Design review of the part built by this model. Coordinates are the model's own, in mm. Give positions to 0.01 mm unless a question says otherwise; leave off trailing zeros. Loops run counter-clockwise (first coordinate to the right, second up) from the corner with the lowest first, then second, coordinate; pieces in that order, holes last.
from build123d import *

# Parameters (mm, degrees)
SKETCH_1_R      = 1.6
EXTRUDE_2_DEPTH = 2.5
SKETCH_2_R      = 1.6
EXTRUDE_4_DEPTH = 2.5


with BuildPart() as part:
    # 草图1 → 凸台-拉伸2 (new body)
    with BuildSketch(Plane.XY):
        with BuildLine():
            Line((-4.793926247, 2), (8.206073753, 2))
            ThreePointArc((8.206073753, 2), (10.206073753, 0), (8.206073753, -2))
            Line((8.206073753, -2), (-4.793926247, -2))
            ThreePointArc((-4.793926247, -2), (-6.793926247, 0), (-4.793926247, 2))
        make_face()
        with Locations((-4.793926247, 0)):
            Circle(SKETCH_1_R, mode=Mode.SUBTRACT)
        with Locations((8.206073753, 0)):
            Circle(SKETCH_1_R, mode=Mode.SUBTRACT)
    extrude(amount=EXTRUDE_2_DEPTH)

    # 草图2 → 凸台-拉伸4 (add)
    with BuildSketch(Plane(origin=(0, 0, 0), x_dir=(-1, 0, 0), z_dir=(0, 0, -1))):
        with BuildLine():
            Line((-8.206073753, 2.5), (4.793926247, 2.5))
            ThreePointArc((4.793926247, 2.5), (7.293926247, 0), (4.793926247, -2.5))
            Line((4.793926247, -2.5), (-8.206073753, -2.5))
            ThreePointArc((-8.206073753, -2.5), (-10.706073753, 0), (-8.206073753, 2.5))
        make_face()
        with Locations(Location((4.793926247, 0, 0), (0, 0, 180))):
            Circle(SKETCH_2_R, mode=Mode.SUBTRACT)
        with Locations(Location((-8.206073753, 0, 0), (0, 0, 180))):
            Circle(SKETCH_2_R, mode=Mode.SUBTRACT)
    extrude(amount=-EXTRUDE_4_DEPTH)


solid = part.part
Q1. Wall thickness on line 1 (X direction, y = 1.1, z = 1.35); line 2 (Y direction, x = 8.25, z = 2.15); line 3 (X direction, y = 1.4, z = 0.45): over which ranges is each line inside the solid? List them lowest first.
Results:
line 1: x = -7.04 to -5.96, -3.63 to 7.04, 9.37 to 10.45
line 2: y = -2.5 to -1.6, 1.6 to 2.5
line 3: x = -6.87 to -5.57, -4.02 to 7.43, 8.98 to 10.28
Q2. Insertion check: pin 1 (3 mm diameter, centred on x = -4.79, y = 0, fed in from -Z). The pin has a flat end and moves straight along its axis. Give the tip position at first contact, or say it passes through.
Results:
pin 1: passes through
Q3. Take a section at A-A (z = 2). Give the boundary of the cut face in (x, y), plus the area to 4 significant figures.
Results:
outline: (-4.79, -2.5) - (8.21, -2.5) arc R2.5 ccw to (8.21, 2.5) - (-4.79, 2.5) arc R2.5 ccw to start; hole circle Ø3.2 at (-4.79, 0); hole circle Ø3.2 at (8.21, 0)
area: 68.55 mm2
Q4. Take a section at D-D (y = -1.95). Give the boundary of the cut face in (x, z), plus the area to 3 significant figures.
Results:
outline: (-6.36, 0) - (9.77, 0) - (9.77, 2.5) - (-6.36, 2.5) - close
area: 40.3 mm2
Q5. Take a section at B-B (x = 7). Give the boundary of the cut face in (y, z).
Results:
outline: (-2.5, 0) - (-1.05, 0) - (-1.05, 2.5) - (-2.5, 2.5) - close; (1.05, 0) - (2.5, 0) - (2.5, 2.5) - (1.05, 2.5) - close
Q6. Take a section at C-C (y = 0). Give the boundary of the cut face in (x, z), plus the area to 3 significant figures.
Results:
outline: (-7.29, 0) - (-6.39, 0) - (-6.39, 2.5) - (-7.29, 2.5) - close; (-3.19, 0) - (6.61, 0) - (6.61, 2.5) - (-3.19, 2.5) - close; (9.81, 0) - (10.71, 0) - (10.71, 2.5) - (9.81, 2.5) - close
area: 29.0 mm2
Q7. Draft analysis for pull direction Y (two halves, no side actions). For faces 1 (the face through (2, 2.5, 1)), 2 (the face through (9.732, 0.481, 1.232)), 3 (the face through (-7.293, 0.055, 1.232)), state which applies: pulls with the +Y half, pulls with the -Y half, needs draft (parallel to the pull), parting line crosses it, or undercut.
Results:
face 1: pulls with the +Y half
face 2: undercut
face 3: parting line crosses it
